Source: CAD feature listing. Evaluate the final solid. Frame: model axes, mm. Face numbers are marked on the shaded views. Coordinates: 2 decimals unless noted, no trailing zeros. Loops run counter-clockwise (first coordinate to the right, second up) from the corner with the lowest first, then second, coordinate; pieces in that order, holes last.
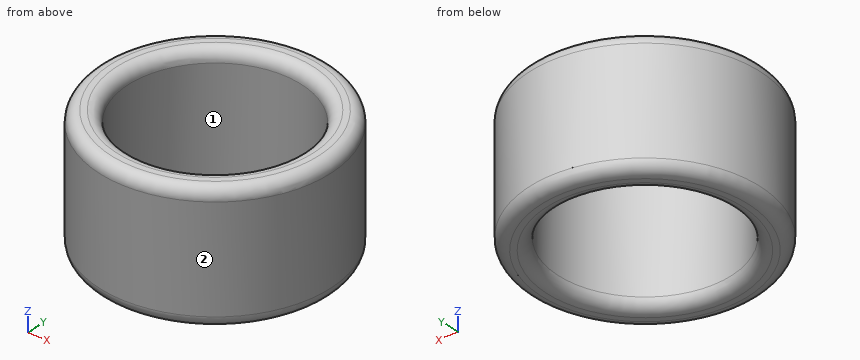
```python
from build123d import *

# Parameters (mm, degrees)
F0_R     = 10
F0_R_2   = 7.5
F1_DEPTH = 11
F2_R     = 1


with BuildPart() as f1:
    # F0 (on Top) → F1 (new body)
    with BuildSketch(Plane.XY):
        Circle(F0_R)
        Circle(F0_R_2, mode=Mode.SUBTRACT)
    extrude(amount=F1_DEPTH)

    # F2
    f2_edges = [f1.edges().sort_by_distance(p)[0] for p in [
        (7.5, 0, 5.5),
        (-7.5, 0, 0),
        (-7.5, 0, 11),
        (-10, 0, 11),
        (-10, 0, 0),
    ]]
    fillet(f2_edges, radius=F2_R)


solid = f1.part
```
Q1. Section query A-A on y = 0. Return the cut outline in (x, z).
Q2. Material intervals for line 1 along Y through (x, z) = (0, 7.25); line 2 along Y through (x, z) = (-6, 4.25); line 3 along X through (y, z) = (-6.5, 7.5), sorted ascending.
Q3. First-contact query: pin 1 Ø1 at (x, z) = (5.5, 5) entering from -Y; pin 2 Ø1 at (x, z) = (-7, 9.5) entering from +Y; pin 3 Ø4 at (y, z) = (4.5, 2) entering from -X. Flat tips, straight axial feed; report the tip coordinate or a pass-through.
Q4. Draft query along Y for the marked faces 1 and 2. Return one class per face: released by +Y, released by -Y, zero draft, split by the parting line, or undercut.
Q5. Section query C-C on z = 9.5. Return the cut outline in (x, y), then the cut area to 3 significant figures.
Resolved:
1. outline: (-10, 1) arc R1 ccw to (-9, 0) - (-8.5, 0) arc R1 ccw to (-7.5, 1) - (-7.5, 10) arc R1 ccw to (-8.5, 11) - (-9, 11) arc R1 ccw to (-10, 10) - close; (7.5, 1) arc R1 ccw to (8.5, 0) - (9, 0) arc R1 ccw to (10, 1) - (10, 10) arc R1 ccw to (9, 11) - (8.5, 11) arc R1 ccw to (7.5, 10) - close
2. line 1: y = -10 to -7.5, 7.5 to 10
2. line 2: y = -8 to -4.5, 4.5 to 8
2. line 3: x = -7.6 to -3.74, 3.74 to 7.6
3. pin 1: stops at y = -8.66
3. pin 2: stops at y = 7.6
3. pin 3: stops at x = -9.68
4. face 1: undercut
4. face 2: split by the parting line
5. outline: circle Ø20 at (0, 0); hole circle Ø15 at (0, 0)
5. area: 137 mm2
